Here's the drawing with two shaded views (mm, measured from the low corner). I have some questions. A direction names the side the tool comes from. Coordinates: 2 decimals unless noted, no trailing zeros. Order: outer loops, then holes, each group sorted by start corner. A loop starts at its lowest first (then second) coordinate and runs counter-clockwise, first axis right, second up. Notation, with made-up numbers: (-27, 65) -> (22, 65) arc R13 ccw to (22, 82) -> close; hole circle Ø10 at (-8, -17.5). An arc over 180 degrees is marked (long way). Answer in a Markdown table with one row per item. Add a question column.
1. Imagine slicing it at A-A on y = 5.65. Write out the boundary of the cut face in (x, z), plus the area to 3 significant figures.
2. Will these pins go through, and if not, where does the flat tip stop? pin 1 (2 mm diameter, centred on y = 3.5, z = 4.5, fed in from -X); pin 2 (3.5 mm diameter, centred on y = 6, z = 5, fed in from -X).
3. Imagine slicing it at C-C on z = 10.25. Write out the boundary of the cut face in (x, y).
4. On a 3-axis mill with a long thin cutter (end or side, diameter ignored), from which of +Z, -Z, +X, -X, +Y, -Y can I reach the whole of each face in a straight line? I mean the marked faces 4 and 5. Say none if no direction works.
5. Imagine slicing it at D-D on x = 1.55. Write out the boundary of the cut face in (y, z), plus the area to 3 significant figures.
6. If I drill on line 1 along Y through (x, z) = (2.05, 5.65); line 2 along Y through (x, z) = (0.7, 8); line 3 along X through (y, z) = (6.5, 10.75), over which ranges is the centre line in solid material (lowest first)? Write a range as [from, to].
7. We'd pull the mould along Y, two halves only. Please class the marked faces 1, 2 and 3: pulls with the +Y half, pulls with the -Y half, needs draft (parallel to the pull), parting line crosses it, or undercut.
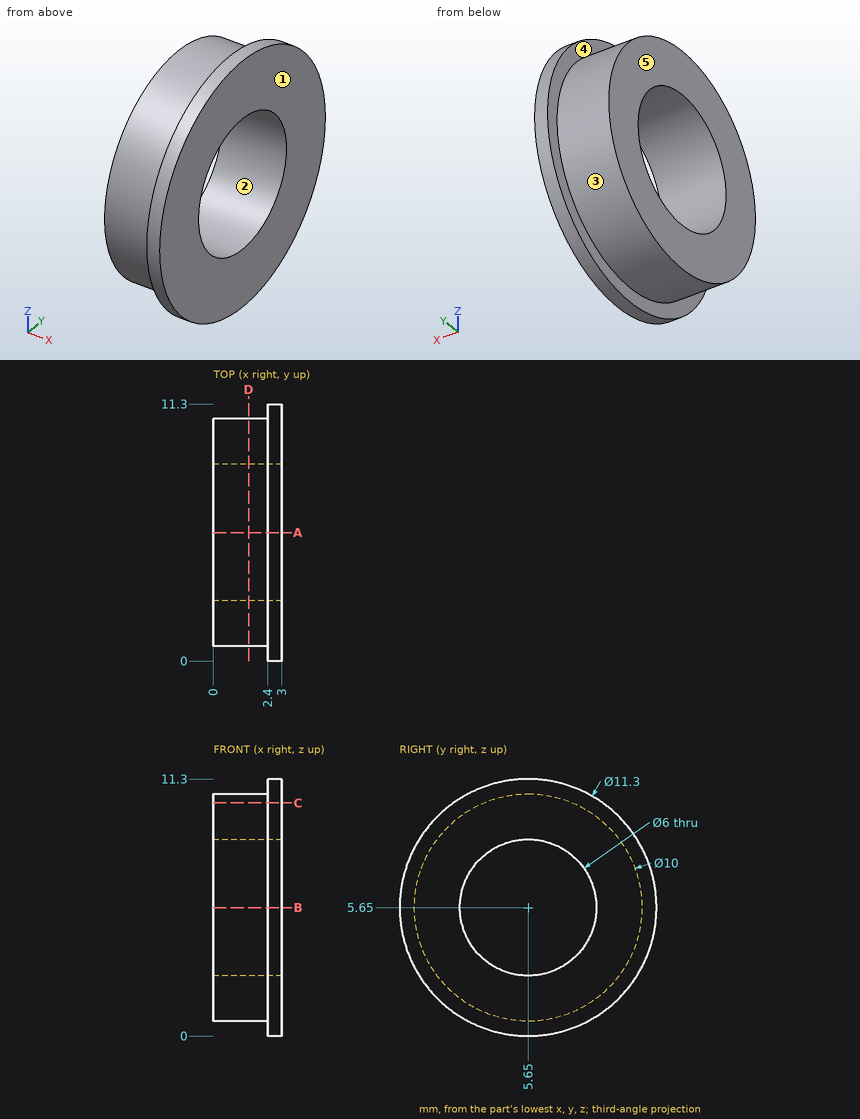
Answers follow:
| question | item | result |
|---|---|---|
| 1 | outline | (0, 0.65) -> (2.4, 0.65) -> (2.4, 0) -> (3, 0) -> (3, 2.65) -> (0, 2.65) -> close; (0, 8.65) -> (3, 8.65) -> (3, 11.3) -> (2.4, 11.3) -> (2.4, 10.65) -> (0, 10.65) -> close |
| 1 | area | 12.8 mm² |
| 2 | pin 1 | stops at x = 0 |
| 2 | pin 2 | passes through |
| 3 | outline | (0, 3.69) -> (2.4, 3.69) -> (2.4, 2.37) -> (3, 2.37) -> (3, 8.93) -> (2.4, 8.93) -> (2.4, 7.61) -> (0, 7.61) -> close |
| 4 | face 4 | -X |
| 4 | face 5 | +Z, -Z, -X, +Y, -Y |
| 5 | outline | circle Ø10 at (5.65, 5.65); hole circle Ø6 at (5.65, 5.65) |
| 5 | area | 50.3 mm² |
| 6 | line 1 | y = [0.65, 2.65], [8.65, 10.65] |
| 6 | line 2 | y = [1.24, 3.79], [7.51, 10.06] |
| 6 | line 3 | x = [2.4, 3] |
| 7 | face 1 | needs draft |
| 7 | face 2 | undercut |
| 7 | face 3 | parting line crosses it |
